Check sheet for the modelled part. Datum: model origin and axes. Units: mm. Face numbers are marked on the shaded views. Round coordinates to 2 decimals unless told otherwise and drop trailing zeros. Order: outer loops, then holes, each group sorted by start corner. A loop starts at its lowest first (then second) coordinate and runs counter-clockwise, first axis right, second up. Notation, with made-up numbers: (76, 74.25) -> (86, 74.25) arc R14 ccw to (86, 100.25) -> close; hole circle Ø8 at (76, 82.5). An arc over 180 degrees is marked (long way). Answer in a Markdown table with one row per item.
```python
from build123d import *

# Parameters (mm, degrees)
SKETCH_1_W          = 40
SKETCH_1_H          = 60
SKETCH_1_R          = 1.5
EXTRUDE_1_DEPTH     = 6
SKETCH_2_R          = 3
CUT_EXTRUDE_1_DEPTH = 3
FILLET_1_R          = 3
CHAMFER_1_SIZE      = 1.6
SKETCH_3_R          = 8.5
CUT_EXTRUDE_2_DEPTH = 37.551333765
SKETCH_4_R          = 11.5
SKETCH_4_R_2        = 8.5
EXTRUDE_2_DEPTH     = 6


with BuildPart() as part:
    # 草圖1 → 填料-伸長1 (new body)
    with BuildSketch(Plane.XY):
        Rectangle(SKETCH_1_W, SKETCH_1_H)
        with Locations((-10, 23)):
            Circle(SKETCH_1_R, mode=Mode.SUBTRACT)
        with Locations(Location((10, 23, 0), (0, 0, 180))):
            Circle(SKETCH_1_R, mode=Mode.SUBTRACT)
        with Locations((10, -23)):
            Circle(SKETCH_1_R, mode=Mode.SUBTRACT)
        with Locations(Location((-10, -23, 0), (0, 0, 180))):
            Circle(SKETCH_1_R, mode=Mode.SUBTRACT)
    extrude(amount=EXTRUDE_1_DEPTH)

    # 草圖2 → 除料-伸長1 (cut)
    with BuildSketch(Plane.XY.offset(6)):
        with Locations((-10, 23)):
            Circle(SKETCH_2_R)
        with Locations((10, 23)):
            Circle(SKETCH_2_R)
        with Locations((10, -23)):
            Circle(SKETCH_2_R)
        with Locations((-10, -23)):
            Circle(SKETCH_2_R)
    extrude(amount=-CUT_EXTRUDE_1_DEPTH, mode=Mode.SUBTRACT)

    # 圓角1
    fillet_1_edges = [part.edges().sort_by_distance(p)[0] for p in [
        (-20, 30, 3),
        (20, 30, 3),
        (20, -30, 3),
        (-20, -30, 3),
    ]]
    fillet(fillet_1_edges, radius=FILLET_1_R)

    # 導角1
    chamfer_1_edges = [part.edges().sort_by_distance(p)[0] for p in [
        (0, -30, 6),
        (-20, 0, 6),
        (20, 0, 6),
        (0, 30, 6),
        (19.121320344, 29.121320344, 6),
        (-19.121320344, 29.121320344, 6),
        (19.121320344, -29.121320344, 6),
        (-19.121320344, -29.121320344, 6),
    ]]
    chamfer(chamfer_1_edges, length=CHAMFER_1_SIZE)

    # 草圖3 → 除料-伸長2 (cut, through all)
    with BuildSketch(Plane.XY.offset(6)):
        Circle(SKETCH_3_R)
    extrude(amount=-CUT_EXTRUDE_2_DEPTH, mode=Mode.SUBTRACT)

    # 草圖4 → 填料-伸長2 (add)
    with BuildSketch(Plane(origin=(0, 0, 0), x_dir=(-1, 0, 0), z_dir=(0, 0, -1))):
        with Locations(Location((0, 0, 0), (0, 0, 180))):
            Circle(SKETCH_4_R)
        with Locations(Location((0, 0, 0), (0, 0, 180))):
            Circle(SKETCH_4_R_2, mode=Mode.SUBTRACT)
    extrude(amount=EXTRUDE_2_DEPTH)


solid = part.part
```
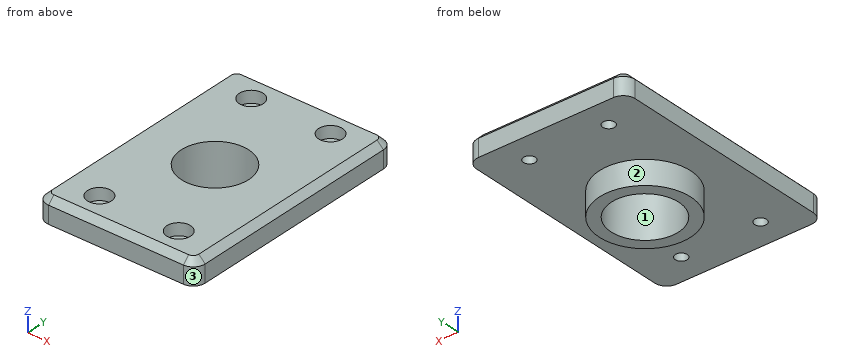
(1) Section check A-A on y = 23. Record the boundary of the cut face in (x, z).
Solutions:
| item | result |
|---|---|
| outline | (-20, 0) -> (-11.5, 0) -> (-11.5, 3) -> (-13, 3) -> (-13, 6) -> (-18.4, 6) -> (-20, 4.4) -> close; (-8.5, 0) -> (8.5, 0) -> (8.5, 3) -> (7, 3) -> (7, 6) -> (-7, 6) -> (-7, 3) -> (-8.5, 3) -> close; (11.5, 0) -> (20, 0) -> (20, 4.4) -> (18.4, 6) -> (13, 6) -> (13, 3) -> (11.5, 3) -> close |
(2) Section check D-D on y = 0. Record the boundary of the cut face in (x, z).
Solutions:
| item | result |
|---|---|
| outline | (-20, 0) -> (-11.5, 0) -> (-11.5, -6) -> (-8.5, -6) -> (-8.5, 6) -> (-18.4, 6) -> (-20, 4.4) -> close; (8.5, -6) -> (11.5, -6) -> (11.5, 0) -> (20, 0) -> (20, 4.4) -> (18.4, 6) -> (8.5, 6) -> close |
(3) Draft check along Y on the marked faces 1, 2 and 3. Enter one of: pulls with the +Y half, pulls with the -Y half, needs draft (parallel to the pull), parting line crosses it, or undercut.
Solutions:
| item | result |
|---|---|
| face 1 | undercut |
| face 2 | parting line crosses it |
| face 3 | pulls with the -Y half |
(4) Section check C-C on x = 0. Record the boundary of the cut face in (y, z).
Solutions:
| item | result |
|---|---|
| outline | (-30, 0) -> (-11.5, 0) -> (-11.5, -6) -> (-8.5, -6) -> (-8.5, 6) -> (-28.4, 6) -> (-30, 4.4) -> close; (8.5, -6) -> (11.5, -6) -> (11.5, 0) -> (30, 0) -> (30, 4.4) -> (28.4, 6) -> (8.5, 6) -> close |
(5) Section check B-B on z = 3.75. Record the boundary of the cut face in (x, y), plus the area to 3 significant figures.
Solutions:
| item | result |
|---|---|
| outline | (-20, -27) arc R3 ccw to (-17, -30) -> (17, -30) arc R3 ccw to (20, -27) -> (20, 27) arc R3 ccw to (17, 30) -> (-17, 30) arc R3 ccw to (-20, 27) -> close; hole circle Ø6 at (-10, -23); hole circle Ø6 at (-10, 23); hole circle Ø17 at (0, 0); hole circle Ø6 at (10, -23); hole circle Ø6 at (10, 23) |
| area | 2,050 mm^2 |
(6) Depth check by flat-ended pin: pin 1 Ø5.5 at (x, y) = (-10, 23) entering from -Z; pin 2 Ø1.8 at (x, y) = (8.5, -23.5) entering from +Z; pin 3 Ø2 at (x, z) = (13, -3.5) entering from +Y. Enter the tip coordinate at first touch or a pass-through.
Solutions:
| item | result |
|---|---|
| pin 1 | z = 0 |
| pin 2 | z = 3 |
| pin 3 | through |
(7) Scan lines: probe 1 along Y at (x, z) = (-10, 1.2); probe 2 along Y at (x, z) = (-10, 4.3); probe 3 along X at (y, z) = (23, 2.05). Record each from-to range of solid material in increasing order. Write a range as from..to.
Solutions:
| item | result |
|---|---|
| probe 1 | -30..-24.5, -21.5..21.5, 24.5..30 |
| probe 2 | -30..-26, -20..20, 26..30 |
| probe 3 | -20..-11.5, -8.5..8.5, 11.5..20 |
